Geometry: final body of the model. Coordinates: model frame, mm. A direction names the side the tool comes from. Give positions to 0.01 mm unless a question says otherwise; leave off trailing zeros. Loops run counter-clockwise (first coordinate to the right, second up) from the corner with the lowest first, then second, coordinate; pieces in that order, holes last. Notation, with made-up numbers: (53, -38.75) -> (107, -38.75) arc R30 ccw to (107, -3.75) -> close; hole circle Ø9 at (72.25, 63). An arc over 180 degrees is marked (long way). Answer in a Markdown table with one row per item. Add a question column.
1) Section query A-A (x = 48.5). Return the cut outline in (y, z), plus the area to 3 significant figures.
2) Access query for faces 1 (the flat face through (0, 0, 0)), 2 (the cylindrical face through (40.97, -27.7, -3.64)). Directions: +Z, -Z, +X, -X, +Y, -Y. A direction counts if a zero-diameter tool reaches every point of the face in a straight line with its end or side. Return the directions, or none.
3) First-contact query: P1, Ø5, axis at x = 33.5, y = -6.5, coming from the -Z side; P2, Ø1, axis at y = 13, z = 12, coming from the +X side; P3, Ø4, axis at x = 52, z = 5.5, coming from the -Y side (3 decimals). Flat tips, straight axial feed; report the tip coordinate or a pass-through.
4) Section query B-B (x = 11). Return the cut outline in (y, z).
5) Line query: line 1 (Z direction, x = 18, y = -0.5); line 2 (Z direction, x = 45, y = 16.5); line 3 (X direction, y = 7.5, z = -5). Output: solid intervals per line, ascending. Write a range as from..to.
6) Draft query along X for faces 3 (the cylindrical face through (47.73, -27.7, -3.64)), 4 (the cylindrical face through (16.279, -13.546, 8.636)), 5 (the conical face through (33.39, 10.126, -13.206)), 6 (the flat face through (52.832, -28, -4)). Return one class per face: +X half, -X half, draft (parallel to the pull), parting line (faces both ways), or undercut.
```python
from build123d import *


with BuildPart() as part:
    # Sketch1 → Revolve4 (revolve)
    with BuildSketch(Plane.XY, mode=Mode.PRIVATE) as revolve4_sk:
        with BuildLine():
            Line((52.832, 0), (52.832, 27.94))
            Line((52.832, 27.94), (42.774202723, 27.94))
            ThreePointArc((42.774202723, 27.94), (42.04078305, 28.673419673), (41.307363376, 27.94))
            Line((41.307363376, 27.94), (40.64, 27.94))
            Line((40.64, 27.94), (33.02, 16.064574588))
            Line((33.02, 16.064574588), (0, 16.064574588))
            Line((0, 16.064574588), (0, 0))
            Line((0, 0), (52.832, 0))
        make_face()
    revolve(revolve4_sk.sketch.rotate(Axis((-76.840094259, 0, 0), (1, 0, 0)), 90), axis=Axis((-76.840094259, 0, 0), (1, 0, 0)))

    # Sketch11 → Revolve7 (revolve)
    with BuildSketch(Plane.XY):
        with BuildLine():
            Line((52.832, 27.94), (52.832, -0.357740308))
            Line((52.832, -0.357740308), (59.182, -0.357740308))
            ThreePointArc((59.182, -0.357740308), (57.575003167, 14.14298904), (52.832, 27.94))
        make_face()
    revolve(axis=Axis((52.832, -0.357740308, 0), (1, 0, 0)))


solid = part.part
```
Evaluation:
| question | item | result |
|---|---|---|
| 1 | outline | circle Ø55.88 at (0, 0) |
| 1 | area | 2,450 mm² |
| 2 | face 1 | +Z, -Z, -X, +Y, -Y |
| 2 | face 2 | -X |
| 3 | P1 | z = -19.74 |
| 3 | P2 | x = 56.84 |
| 3 | P3 | y = -28.415 |
| 4 | outline | circle Ø32.13 at (0, 0) |
| 5 | line 1 | -16.06..16.06 |
| 5 | line 2 | -22.55..22.55 |
| 5 | line 3 | 0..58.52 |
| 6 | face 3 | undercut |
| 6 | face 4 | draft |
| 6 | face 5 | -X half |
| 6 | face 6 | undercut |
